CAD build for the part. Positions are in the model's coordinates, mm. A direction names the side the tool comes from. Give positions to 0.01 mm unless a question says otherwise; leave off trailing zeros. Answer as a JSON object with one key per item and string values.
from build123d import *

# Parameters (mm, degrees)
CUT_EXTRUDE1_DEPTH      = 5.5626
CUT_EXTRUDE1_DEPTH_BACK = 5.5626
SKETCH2_W               = 1.524
SKETCH2_H               = 23.8125
SKETCH5_W               = 11.1252
SKETCH5_H               = 1.9558
SKETCH6_W               = 11.1252
SKETCH6_H               = 1.9558


with BuildPart() as part:
    # Sketch1 → Revolve1 (revolve)
    with BuildSketch(Plane.XY, mode=Mode.PRIVATE) as revolve1_sk:
        Polygon((-5.5626, 6.858), (-5.0546, 6.35), (5.0546, 6.35), (5.5626, 6.858), (5.5626, 13.7795), (5.0546, 14.2875), (-5.0546, 14.2875), (-5.5626, 13.7795), align=None)
    revolve(revolve1_sk.sketch.rotate(Axis((5.5626, 0, 0), (-1, 0, 0)), 270), axis=Axis((5.5626, 0, 0), (-1, 0, 0)))

    # Sketch2 → Cut-Extrude1 (cut, two sides: drawn at the far end of the back side and taken through both)
    with BuildSketch(Plane(origin=(0, 0, 0), x_dir=(0, 0, -1), z_dir=(1, 0, 0)).offset(-CUT_EXTRUDE1_DEPTH_BACK)):
        with Locations((0, -2.38125)):
            Rectangle(SKETCH2_W, SKETCH2_H)
    extrude(amount=CUT_EXTRUDE1_DEPTH + CUT_EXTRUDE1_DEPTH_BACK, mode=Mode.SUBTRACT)

    # Sketch3 → Cut-Revolve1 (revolve, cut)
    with BuildSketch(Plane(origin=(0, 0, 0), x_dir=(0, 0, -1), z_dir=(1, 0, 0)), mode=Mode.PRIVATE) as cut_revolve1_sk:
        Polygon((-14.2875, -10.3124), (-14.2875, -6.35), (-3.5814, -6.35), (-3.5814, -8.0264), (0, -8.0264), (0, -10.3124), align=None)
    revolve(cut_revolve1_sk.sketch.rotate(Axis((0, -10.3124, 0), (0, 0, 1)), 270), axis=Axis((0, -10.3124, 0), (0, 0, 1)), mode=Mode.SUBTRACT)

    # Sketch4 → Cut-Revolve2 (revolve, cut)
    with BuildSketch(Plane(origin=(0, 0, 0), x_dir=(0, 0, -1), z_dir=(1, 0, 0)), mode=Mode.PRIVATE) as cut_revolve2_sk:
        Polygon((0.762, -10.3124), (0.762, -8.2296), (1.1938, -8.6614), (16.2306, -8.6614), (16.2306, -10.3124), align=None)
    revolve(cut_revolve2_sk.sketch.rotate(Axis((0, -10.3124, -16.2306), (0, 0, 1)), 270), axis=Axis((0, -10.3124, -16.2306), (0, 0, 1)), mode=Mode.SUBTRACT)

    # Sketch5 → Cut-Revolve3 (revolve, cut)
    with BuildSketch(Plane(origin=(0, 0, 0), x_dir=(1, 0, 0), z_dir=(0, 1, 0)), mode=Mode.PRIVATE) as cut_revolve3_sk:
        with Locations((0, 11.303)):
            Rectangle(SKETCH5_W, SKETCH5_H)
    revolve(cut_revolve3_sk.sketch.rotate(Axis((5.5626, 0, -10.3251), (-1, 0, 0)), 180), axis=Axis((5.5626, 0, -10.3251), (-1, 0, 0)), mode=Mode.SUBTRACT)

    # Sketch6 → Cut-Revolve4 (revolve, cut)
    with BuildSketch(Plane(origin=(0, 0, 0), x_dir=(1, 0, 0), z_dir=(0, 1, 0)), mode=Mode.PRIVATE) as cut_revolve4_sk:
        with Locations((0, -9.3472)):
            Rectangle(SKETCH6_W, SKETCH6_H)
    revolve(cut_revolve4_sk.sketch.rotate(Axis((5.5626, 0, 10.3251), (-1, 0, 0)), 180), axis=Axis((5.5626, 0, 10.3251), (-1, 0, 0)), mode=Mode.SUBTRACT)


solid = part.part
(1) Saw through at A-A, the plane x = 0. State how many separate pieces and enclosed holes the cut face has, and give its area (3 significant figures).
Answer key:
{"separate pieces": "3", "enclosed holes": "2", "area": "386 mm²"}
(2) Probe L1, parallel to Z at x = -3, y = 0.25; L2, parallel to Z at x = 4.5, y = 0.75; L3, parallel to Y at x = 0, z = 2.7. List the from-to ranges inside material, lowest first. Write a range as [from, to].
Answer key:
{"L1": "z = [-14.29, -12.26], [-8.39, -6.35], [6.35, 8.39], [12.26, 14.29]", "L2": "z = [-14.27, -12.13], [-8.52, -6.31], [6.31, 8.52], [12.13, 14.27]", "L3": "y = [-14.03, -12.6], [-8.03, -5.75], [5.75, 14.03]"}
(3) Flat gauge pins, fed straight in: P1, Ø6, axis at x = 1, y = 11, coming from the -Z side; P2, Ø4, axis at x = 4.5, z = -4, coming from the -Y side; P3, Ø6.5, axis at y = 0, z = -10.33, coming from the +X side; P4, Ø2.5, axis at x = -1.5, y = -10, coming from the +Z side. Where does each tip first touch, or does it go through?
Answer key:
{"P1": "stops at z = -11.84", "P2": "stops at y = -14.15", "P3": "stops at x = 5.56", "P4": "stops at z = 3.58"}
(4) 3-axis set-ups, long thin cutter, end or side, ignore diameter. For faces 1 (the face through (-1.814, -11.703, 2.152)), 2 (the face through (-5.192, 0.133, -6.486)), 3 (the face through (2.4, -10.3, -0.762)): which of +Z, -Z, +X, -X, +Y, -Y reach the whole face in a straight line?
Answer key:
{"face 1": "+Z", "face 2": "-X", "face 3": "+X, -X, -Y"}
(5) Pull direction Y, two halves, no side cores. Call faces 4 (the face through (5.563, 3.3, 6.3)), 5 (the face through (5.199, 0.133, -6.493)), 6 (the face through (5.42, 13.91, 0.6)): pulls with the +Y half, pulls with the -Y half, needs draft (parallel to the pull), parting line crosses it, or undercut.
Answer key:
{"face 4": "needs draft", "face 5": "undercut", "face 6": "parting line crosses it"}
